Here's how the part is built. I have some questions about the finished solid (model axes, mm). Face numbers are marked on the shaded views. A direction names the side the tool comes from. Round coordinates to 2 decimals unless told otherwise and drop trailing zeros. Loops run counter-clockwise (first coordinate to the right, second up) from the corner with the lowest first, then second, coordinate; pieces in that order, holes last. Notation, with made-up numbers: M -25,83.5 L -2,83.5 A31 cw -2,121.5 Z; hole C 11,30.5 d3. An arc over 180 degrees is marked long. Write item = value, one per line. Start each with the question number.
from build123d import *

# Parameters (mm, degrees)
CHAMFER1_SIZE = 2
CHAMFER2_SIZE = 1


with BuildPart() as part:
    # Sketch1 → Revolve1 (revolve)
    with BuildSketch(Plane.XY, mode=Mode.PRIVATE) as revolve1_sk:
        Polygon((0, 0), (30, 0), (30, 8), (0, 8), (0, 7), (-2, 7), (-2, 11.5), (-66, 11.5), (-66, 5), (-68, 5), (-68, 6), (-90, 6), (-90, 0), (-68, 0), (-66, 0), (-2, 0), align=None)
    revolve(revolve1_sk.sketch.rotate(Axis((-68, 0, 0), (-1, 0, 0)), 90), axis=Axis((-68, 0, 0), (-1, 0, 0)))

    # Chamfer1
    chamfer1_edges = [part.edges().sort_by_distance(p)[0] for p in [
        (30, 0, 8),
    ]]
    chamfer(chamfer1_edges, length=CHAMFER1_SIZE)

    # Chamfer2
    chamfer2_edges = [part.edges().sort_by_distance(p)[0] for p in [
        (-90, 0, 6),
    ]]
    chamfer(chamfer2_edges, length=CHAMFER2_SIZE)


solid = part.part
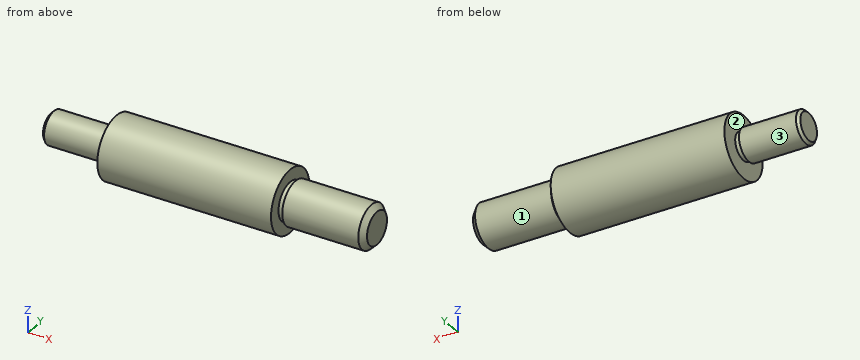
Item 1: Please list where these lines run through material, in increasing order: line 1 (X direction, y = -5.5, z = -9.25); line 2 (Y direction, x = -71.5, z = 0); line 3 (Y direction, x = -55, z = -1.25). Write a range as [from, to].
Item 2: I want a section at D-D, the plane x = -47.5. List the corners of the cut face in (y, z) for me.
Item 3: I want a section at C-C, the plane x = -74. List the corners of the cut face in (y, z) for me, then the cut area to 3 significant figures.
Item 4: Will these pins go through, and if not, where does the flat tip stop? pin 1 Ø4 at (x, y) = (-47.5, 7.5) entering from -Z; pin 2 Ø3 at (x, y) = (-32.5, -2) entering from +Z; pin 3 Ø8 at (y, z) = (7, -8) entering from +X.
Item 5: For the marked faces 1, 2 and 3, which set-ups out of +Z, -Z, +X, -X, +Y, -Y let a thin tool reach every point of the face, with its end or its side?
Item 6: I want a section at A-A, the plane z = 0. List the corners of the cut face in (x, y) for me.
Worked out:
q1.line_1 = [-66, -2]
q1.line_2 = [-6, 6]
q1.line_3 = [-11.43, 11.43]
q2.outline = C 0,0 d23
q3.outline = C 0,0 d12
q3.area = 113 mm2
q4.pin_1 = -10.1
q4.pin_2 = 11.49
q4.pin_3 = 29.37
q5.face_1 = +X
q5.face_2 = none
q5.face_3 = -X
q6.outline = M -90,-5 L -89,-6 L -68,-6 L -68,-5 L -66,-5 L -66,-11.5 L -2,-11.5 L -2,-7 L 0,-7 L 0,-8 L 28,-8 L 30,-6 L 30,6 L 28,8 L 0,8 L 0,7 L -2,7 L -2,11.5 L -66,11.5 L -66,5 L -68,5 L -68,6 L -89,6 L -90,5 Z
